Job drawing, mm, ordinate dimensions from the low corner. One solid piece. Coordinates: 2 decimals unless noted, no trailing zeros. Order: outer loops, then holes, each group sorted by start corner. A loop starts at its lowest first (then second) coordinate and runs counter-clockwise, first axis right, second up. Notation, with made-up numbers: (83.25, 41.25) - (107.25, 41.25) arc R20 cw to (107.25, 62.25) - close; hole circle Ø3 at (-9, 57.5). An arc over 180 degrees is marked (long way). Return JSON: item names as keys, results as strings.
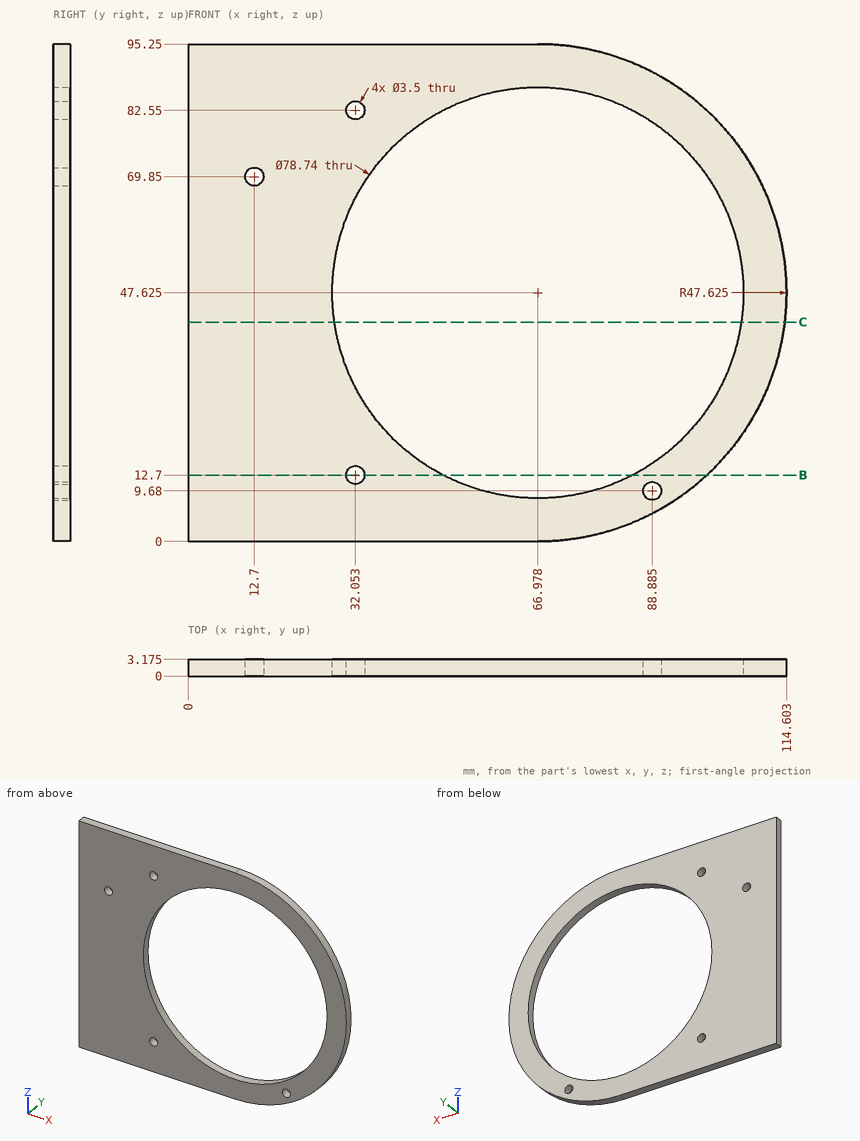
1. Cut at C-C on z = 42. Give the cut face in (x, y) (1 decimal).
Check values:
{"outline": "(0, 0) - (28, 0) - (28, 3.2) - (0, 3.2) - close; (105.9, 0) - (114.3, 0) - (114.3, 3.2) - (105.9, 3.2) - close"}
2. Probe L1, parallel to X at y = 1.6, z = 13.5 (1 decimal); L2, parallel to Z at x = 89, y = 0.7 (1 decimal); L3, parallel to Z at x = 79, y = 2.4 (1 decimal). List the from-to ranges inside material, lowest first.
Check values:
{"L1": "0 to 30.5, 33.6 to 47.3, 86.6 to 100.2", "L2": "5.4 to 7.9, 11.4 to 15, 80.3 to 89.9", "L3": "1.5 to 10.1, 85.1 to 93.7"}
3. Cut at B-B on z = 12.7. State how many separate pieces and enclosed holes the cut face has, plus the area to 3 significant figures.
Check values:
{"separate pieces": "3", "enclosed holes": "0", "area": "189 mm²"}
